Source: CAD feature listing. Evaluate the final solid. Frame: model axes, mm. A direction names the side the tool comes from. Coordinates: 2 decimals unless noted, no trailing zeros. Order: outer loops, then holes, each group sorted by start corner. A loop starts at its lowest first (then second) coordinate and runs counter-clockwise, first axis right, second up. Notation, with made-up numbers: (-17, 44) -> (38, 44) arc R18 ccw to (38, 66) -> close; hole circle Ø8 at (0, 88). An arc over 180 degrees is marked (long way). Put each result on its own line as item: value.
from build123d import *

# Parameters (mm, degrees)
SKETCH1_R           = 3.65
SKETCH1_R_2         = 1.8
SKETCH1_W           = 6.8
SKETCH1_H           = 6.56
SKETCH1_R_3         = 1.6
SKETCH1_R_4         = 2.6
BOSS_EXTRUDE1_DEPTH = 6.2
CUT_EXTRUDE1_DEPTH  = 7.2
SKETCH3_R           = 0.25
CUT_EXTRUDE2_DEPTH  = 7.2
FILLET1_R           = 1
FILLET2_R           = 0.5


with BuildPart() as part:
    # Sketch1 → Boss-Extrude1 (new body)
    with BuildSketch(Plane.XY):
        with BuildLine():
            Line((0, 5.3), (0, 0))
            Line((0, 0), (74.2, 0))
            Line((74.2, 0), (74.2, 5.3))
            Line((74.2, 5.3), (68, 5.3))
            Line((68, 5.3), (68, 11.5))
            Line((68, 11.5), (74.2, 11.5))
            Line((74.2, 11.5), (74.2, 27))
            Line((74.2, 27), (68, 27))
            Line((68, 27), (68, 33.56))
            Line((68, 33.56), (74.2, 33.56))
            Line((74.2, 33.56), (74.2, 91.4))
            ThreePointArc((74.2, 91.4), (71.271067812, 98.471067812), (64.2, 101.4))
            Line((64.2, 101.4), (10, 101.4))
            ThreePointArc((10, 101.4), (2.928932188, 98.471067812), (0, 91.4))
            Line((0, 91.4), (0, 33.56))
            Line((0, 33.56), (6.2, 33.56))
            Line((6.2, 33.56), (6.2, 27))
            Line((6.2, 27), (0, 27))
            Line((0, 27), (0, 11.5))
            Line((0, 11.5), (6.2, 11.5))
            Line((6.2, 11.5), (6.2, 5.3))
            Line((6.2, 5.3), (0, 5.3))
        make_face()
        with Locations((12.5, 10)):
            Circle(SKETCH1_R, mode=Mode.SUBTRACT)
        with Locations((3.1, 16.28)):
            Circle(SKETCH1_R_2, mode=Mode.SUBTRACT)
        with Locations((11.85, 30.28)):
            Circle(SKETCH1_R_2, mode=Mode.SUBTRACT)
        with Locations((22, 30.28)):
            Rectangle(SKETCH1_W, SKETCH1_H, mode=Mode.SUBTRACT)
        with Locations((37.1, 10)):
            Circle(SKETCH1_R, mode=Mode.SUBTRACT)
        with Locations((61.7, 10)):
            Circle(SKETCH1_R, mode=Mode.SUBTRACT)
        with Locations((71.1, 16.28)):
            Circle(SKETCH1_R_2, mode=Mode.SUBTRACT)
        with Locations((52.2, 30.28)):
            Rectangle(SKETCH1_W, SKETCH1_H, mode=Mode.SUBTRACT)
        with Locations((62.35, 30.28)):
            Circle(SKETCH1_R_2, mode=Mode.SUBTRACT)
        with Locations((12.1, 54.75)):
            Circle(SKETCH1_R_3, mode=Mode.SUBTRACT)
        with Locations((12, 89.4)):
            Circle(SKETCH1_R, mode=Mode.SUBTRACT)
        with Locations((62.1, 54.75)):
            Circle(SKETCH1_R_3, mode=Mode.SUBTRACT)
        with Locations((62.2, 89.4)):
            Circle(SKETCH1_R_4, mode=Mode.SUBTRACT)
    extrude(amount=BOSS_EXTRUDE1_DEPTH)

    # Sketch2 → Cut-Extrude1 (cut, through all)
    with BuildSketch(Plane.XY.offset(6.2)):
        with BuildLine():
            Line((33, 80.4), (41.2, 80.4))
            ThreePointArc((41.2, 80.4), (49.2, 72.4), (41.2, 64.4))
            Line((41.2, 64.4), (33, 64.4))
            ThreePointArc((33, 64.4), (25, 72.4), (33, 80.4))
        make_face()
    extrude(amount=-CUT_EXTRUDE1_DEPTH, mode=Mode.SUBTRACT)

    # Sketch3 → Cut-Extrude2 (cut, through all)
    with BuildSketch(Plane.XY.offset(6.2)):
        with Locations((6.2, 33.56)):
            Circle(SKETCH3_R)
        with Locations((6.2, 27)):
            Circle(SKETCH3_R)
        with Locations((6.2, 11.5)):
            Circle(SKETCH3_R)
        with Locations((6.2, 5.3)):
            Circle(SKETCH3_R)
        with Locations((25.4, 27)):
            Circle(SKETCH3_R)
        with Locations((18.6, 27)):
            Circle(SKETCH3_R)
        with Locations((18.6, 33.56)):
            Circle(SKETCH3_R)
        with Locations((25.4, 33.56)):
            Circle(SKETCH3_R)
        with Locations((48.8, 33.56)):
            Circle(SKETCH3_R)
        with Locations((48.8, 27)):
            Circle(SKETCH3_R)
        with Locations((55.6, 33.56)):
            Circle(SKETCH3_R)
        with Locations((55.6, 27)):
            Circle(SKETCH3_R)
        with Locations((68, 33.56)):
            Circle(SKETCH3_R)
        with Locations((68, 27)):
            Circle(SKETCH3_R)
        with Locations((68, 11.5)):
            Circle(SKETCH3_R)
        with Locations((68, 5.3)):
            Circle(SKETCH3_R)
    extrude(amount=-CUT_EXTRUDE2_DEPTH, mode=Mode.SUBTRACT)

    # Fillet1
    fillet1_edges = [part.edges().sort_by_distance(p)[0] for p in [
        (5.95, 33.56, 3.1),
        (6.2, 33.31, 3.1),
        (6.2, 27.25, 3.1),
        (5.95, 27, 3.1),
        (5.95, 11.5, 3.1),
        (6.2, 11.25, 3.1),
        (6.2, 5.55, 3.1),
        (5.95, 5.3, 3.1),
        (25.4, 27.25, 3.1),
        (25.15, 27, 3.1),
        (18.85, 27, 3.1),
        (18.6, 27.25, 3.1),
        (18.85, 33.56, 3.1),
        (18.6, 33.31, 3.1),
        (25.15, 33.56, 3.1),
        (25.4, 33.31, 3.1),
        (49.05, 33.56, 3.1),
        (48.8, 33.31, 3.1),
        (49.05, 27, 3.1),
        (48.8, 27.25, 3.1),
        (55.35, 33.56, 3.1),
        (55.6, 33.31, 3.1),
        (55.6, 27.25, 3.1),
        (55.35, 27, 3.1),
        (68, 33.31, 3.1),
        (68.25, 33.56, 3.1),
        (68.25, 27, 3.1),
        (68, 27.25, 3.1),
        (68, 11.25, 3.1),
        (68.25, 11.5, 3.1),
        (68.25, 5.3, 3.1),
        (68, 5.55, 3.1),
    ]]
    fillet(fillet1_edges, radius=FILLET1_R)

    # Fillet2
    fillet2_edges = [part.edges().sort_by_distance(p)[0] for p in [
        (74.2, 33.56, 3.1),
        (74.2, 27, 3.1),
        (74.2, 11.5, 3.1),
        (74.2, 5.3, 3.1),
        (74.2, 0, 3.1),
        (0, 0, 3.1),
        (0, 5.3, 3.1),
        (0, 11.5, 3.1),
        (0, 27, 3.1),
        (0, 33.56, 3.1),
    ]]
    fillet(fillet2_edges, radius=FILLET2_R)


solid = part.part
1. Cut plane A-A on x = 23. Output: boundary loops of the cut face in (y, z).
Numbers:
outline: (0, 0) -> (27, 0) -> (27, 6.2) -> (0, 6.2) -> close; (33.56, 0) -> (101.4, 0) -> (101.4, 6.2) -> (33.56, 6.2) -> close
2. Cut plane B-B on y = 72.4. Output: boundary loops of the cut face in (x, z), plus the area to 3 significant figures.
Numbers:
outline: (0, 0) -> (25, 0) -> (25, 6.2) -> (0, 6.2) -> close; (49.2, 0) -> (74.2, 0) -> (74.2, 6.2) -> (49.2, 6.2) -> close
area: 310 mm2
3. Set-up query: faces 1 (the flat face through (3, 5.3, 3)), 2 (the flat face through (71, 27, 3)), 3 (the flat face through (52, 33.56, 3)). Return all of +Z, -Z, +X, -X, +Y, -Y with unobstructed straight access to the full face (end or side cutting, diameter ignored); none if empty.
Numbers:
face 1: +Z, -Z, -X
face 2: +Z, -Z, +X
face 3: +Z, -Z
4. Pull-direction query (Y, two-part tool) for faces 4 (the flat face through (0, 63, 3)), 5 (the flat face through (3, 33.56, 3)); classes: pulls with the +Y half, pulls with the -Y half, needs draft (parallel to the pull), parting line crosses it, or undercut.
Numbers:
face 4: needs draft
face 5: undercut
5. Cut plane D-D on y = 30.28. Output: boundary loops of the cut face in (x, z).
Numbers:
outline: (6.2, 0) -> (10.05, 0) -> (10.05, 6.2) -> (6.2, 6.2) -> close; (13.65, 0) -> (18.6, 0) -> (18.6, 6.2) -> (13.65, 6.2) -> close; (25.4, 0) -> (48.8, 0) -> (48.8, 6.2) -> (25.4, 6.2) -> close; (55.6, 0) -> (60.55, 0) -> (60.55, 6.2) -> (55.6, 6.2) -> close; (64.15, 0) -> (68, 0) -> (68, 6.2) -> (64.15, 6.2) -> close
6. First-contact query: pin 1 (1.5 mm diameter, centred on x = 2.5, z = 2.5, fed in from +Y); pin 2 (4.5 mm diameter, centred on x = 12.5, y = 10, fed in from +Z); pin 3 (1.4 mm diameter, centred on y = 9.5, z = 2, fed in from -X). Flat tips, straight axial feed; report the tip coordinate or a pass-through.
Numbers:
pin 1: stops at y = 98.78
pin 2: passes through
pin 3: stops at x = 6.2
7. Ray query, line 1 along X through (y, z) = (54.5, 5.5); line 2 along Y through (x, z) = (62.1, 5); line 3 along Y through (x, z) = (35, 3.75). Return the intervals inside material, ascending.
Numbers:
line 1: x = 0 to 10.52, 13.68 to 60.52, 63.68 to 74.2
line 2: y = 0 to 6.37, 13.63 to 28.5, 32.06 to 53.15, 56.35 to 86.8, 92 to 101.4
line 3: y = 0 to 7.01, 12.99 to 64.4, 80.4 to 101.4
8. Cut plane C-C on x = 37.1. Output: boundary loops of the cut face in (y, z), plus the area to 3 significant figures.
Numbers:
outline: (0, 0) -> (6.35, 0) -> (6.35, 6.2) -> (0, 6.2) -> close; (13.65, 0) -> (64.4, 0) -> (64.4, 6.2) -> (13.65, 6.2) -> close; (80.4, 0) -> (101.4, 0) -> (101.4, 6.2) -> (80.4, 6.2) -> close
area: 484 mm2
